The model under review builds one solid part; all positions refer to its coordinate system, in mm. Coordinates: 2 decimals unless noted, no trailing zeros. Loops run counter-clockwise (first coordinate to the right, second up) from the corner with the lowest first, then second, coordinate; pieces in that order, holes last. Notation, with made-up numbers: (87.25, 79) - (133.25, 79) arc R31 ccw to (133.25, 111) - close; hole circle Ø2 at (49.5, -31). An arc over 180 degrees is marked (long way). Answer in a Markdown table with one row per item. Add a question column.
(1) For P1, Ø1.5, axis at y = -0.5, z = 7.5, coming from the -X side; P2, Ø1.5, axis at x = 6.5, z = -15, coming from the +Y side; P3, Ø2.5, axis at x = 0, z = 9.5, coming from the +Y side; P4, Ø1, axis at y = -2.5, z = -4.5, coming from the -X side, all flat-tipped, find the tip position at first contact; note any pin that passes through.
(2) We need section A-A on x = 0. Write out the cut boundary in (y, z), plus the area to 3 significant figures.
(3) For line 1 along Z through (x, y) = (0, -1.25); line 2 along Z through (x, y) = (14, -2.15); line 3 along Z through (x, y) = (16, -0.35), list the stretches that pass through material, from the lowest coordinate up.
(4) We need section C-C on x = 14. Write out the cut boundary in (y, z), plus the area to 3 significant figures.
(5) We need section D-D on z = 3.5. Write out the cut boundary in (x, y).
(6) We need section B-B on y = -1.05. Give the number of separate pieces and of enclosed holes in the cut face, plus the area to 3 significant figures.
from build123d import *

# Parameters (mm, degrees)
F0_R     = 1.55
F0_R_2   = 1.5
F0_R_3   = 4.25
F1_DEPTH = 3
F2_SIZE  = 1.3


with BuildPart() as f1:
    # F0 (on Front) → F1 (new body)
    with BuildSketch(Plane.XZ):
        with BuildLine():
            Line((-16.5, -6.5), (-19.968726, -6.5))
            ThreePointArc((-19.968726, -6.5), (-14.849242, -14.849242), (-6.5, -19.968726))
            Line((-6.5, -19.968726), (-6.5, -16.5))
            Line((-6.5, -16.5), (0, -16.5))
            Line((0, -16.5), (6.5, -16.5))
            Line((6.5, -16.5), (6.5, -19.968726))
            ThreePointArc((6.5, -19.968726), (14.849242, -14.849242), (19.968726, -6.5))
            Line((19.968726, -6.5), (16.5, -6.5))
            Line((16.5, -6.5), (16.5, 0))
            Line((16.5, 0), (16.5, 6.5))
            Line((16.5, 6.5), (19.968726, 6.5))
            ThreePointArc((19.968726, 6.5), (14.849242, 14.849242), (6.5, 19.968726))
            Line((6.5, 19.968726), (6.5, 16.5))
            Line((6.5, 16.5), (0, 16.5))
            Line((0, 16.5), (-6.5, 16.5))
            Line((-6.5, 16.5), (-6.5, 19.968726))
            ThreePointArc((-6.5, 19.968726), (-12.017667, 17.221373), (-16.5, 12.990381))
            ThreePointArc((-16.5, 12.990381), (-18.520887, 9.898321), (-19.968726, 6.5))
            Line((-19.968726, 6.5), (-16.5, 6.5))
            Line((-16.5, 6.5), (-16.5, 0))
            Line((-16.5, 0), (-16.5, -6.5))
        make_face()
        with Locations((-8.5, -14.722432)):
            Circle(F0_R, mode=Mode.SUBTRACT)
        with Locations((-14.722432, -8.5)):
            Circle(F0_R, mode=Mode.SUBTRACT)
        with Locations((8.5, -14.722432)):
            Circle(F0_R, mode=Mode.SUBTRACT)
        with Locations((0, -9.5)):
            Circle(F0_R_2, mode=Mode.SUBTRACT)
        with Locations((14.722432, -8.5)):
            Circle(F0_R, mode=Mode.SUBTRACT)
        with Locations((-14.722432, 8.5)):
            Circle(F0_R, mode=Mode.SUBTRACT)
        with Locations((-8, 0)):
            Circle(F0_R_2, mode=Mode.SUBTRACT)
        with Locations((-8.5, 14.722432)):
            Circle(F0_R, mode=Mode.SUBTRACT)
        Circle(F0_R_3, mode=Mode.SUBTRACT)
        with Locations((8, 0)):
            Circle(F0_R_2, mode=Mode.SUBTRACT)
        with Locations((0, 9.5)):
            Circle(F0_R_2, mode=Mode.SUBTRACT)
        with Locations((14.722432, 8.5)):
            Circle(F0_R, mode=Mode.SUBTRACT)
        with Locations((8.5, 14.722432)):
            Circle(F0_R, mode=Mode.SUBTRACT)
    extrude(amount=F1_DEPTH)

    # F2
    f2_edges = [f1.edges().sort_by_distance(p)[0] for p in [
        (-1.5, -3, 9.5),
        (-9.5, -3, 0),
        (6.5, -3, 0),
        (-1.5, -3, -9.5),
    ]]
    chamfer(f2_edges, length=F2_SIZE)


solid = f1.part
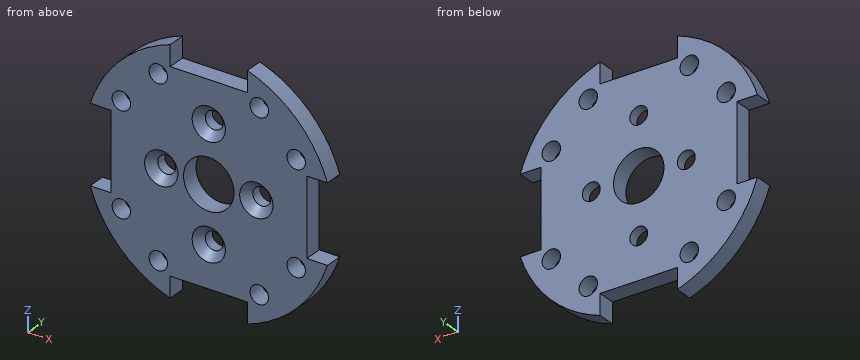
Outcome:
| question | item | result |
|---|---|---|
| 1 | P1 | x = -19.89 |
| 1 | P2 | y = 0 |
| 1 | P3 | through |
| 1 | P4 | x = -16.5 |
| 2 | outline | (-3, -16.5) - (0, -16.5) - (0, -11) - (-1.7, -11) - (-3, -12.3) - close; (-3, -6.7) - (-1.7, -8) - (0, -8) - (0, -4.25) - (-3, -4.25) - close; (-3, 4.25) - (0, 4.25) - (0, 8) - (-1.7, 8) - (-3, 6.7) - close; (-3, 12.3) - (-1.7, 11) - (0, 11) - (0, 16.5) - (-3, 16.5) - close |
| 2 | area | 52.1 mm² |
| 3 | line 1 | -16.5 to -11, -8 to -4.25, 4.25 to 8, 11 to 16.5 |
| 3 | line 2 | -15.65 to -9.87, -7.13 to 7.13, 9.87 to 15.65 |
| 3 | line 3 | -13.6 to -9.38, -7.62 to 7.62, 9.38 to 13.6 |
| 4 | outline | (-3, -15.65) - (0, -15.65) - (0, -9.87) - (-3, -9.87) - close; (-3, -7.13) - (0, -7.13) - (0, 7.13) - (-3, 7.13) - close; (-3, 9.87) - (0, 9.87) - (0, 15.65) - (-3, 15.65) - close |
| 4 | area | 77.5 mm² |
| 5 | outline | (-16.5, -3) - (-2.41, -3) - (-2.41, 0) - (-16.5, 0) - close; (2.41, -3) - (16.5, -3) - (16.5, 0) - (2.41, 0) - close |
| 6 | separate pieces | 1 |
| 6 | enclosed holes | 13 |
| 6 | area | 1,020 mm² |
